Read the model definition and answer for the solid it produces. Units are mm, in the model's axes. A direction names the side the tool comes from. Coordinates: 2 decimals unless noted, no trailing zeros. Write each loop counter-clockwise with the first axis right and the second up, starting at its lowest first coordinate (ties: lowest second). Pieces come first, ordered by that corner, then holes. Notation, with made-up numbers: (-6.5, 45.5) -> (34.5, 45.5) arc R34 ccw to (34.5, 81.5) -> close; hole circle Ø5 at (39.25, 43.25). An arc over 180 degrees is marked (long way). Use CSV: the item, a comma, the result in double quotes.
from build123d import *

# Parameters (mm, degrees)
SKICA1_W                                         = 61
SKICA1_H                                         = 17.5
P_IDAT_VYSUNUT_M1_DEPTH                          = 6
SKICA2_W                                         = 43.1
SKICA2_H                                         = 7.8
P_IDAT_VYSUNUT_M2_DEPTH                          = 20
V_LCOV_ZAHLOUBEN_PRO_M3_ROUBY_S_VNIT_D           = 3.4
V_LCOV_ZAHLOUBEN_PRO_M3_ROUBY_S_VNIT_DEPTH       = 10
V_LCOV_ZAHLOUBEN_PRO_M3_ROUBY_S_VNIT_CBORE_D     = 6.5
V_LCOV_ZAHLOUBEN_PRO_M3_ROUBY_S_VNIT_CBORE_DEPTH = 3.4
V_LCOV_ZAHLOUBEN_PRO_M3_ROUBY_S_VNIT_TIP         = 1.021463052
SKICA5_W                                         = 38.387641765
SKICA5_H                                         = 14.060547141
P_IDAT_VYSUNUT_M3_DEPTH                          = 10
SKICA6_W                                         = 38.387641765
SKICA6_H                                         = 5
P_IDAT_VYSUNUT_M4_DEPTH                          = 1.319108231


with BuildPart() as part:
    # Skica1 → Přidat vysunutím1 (new body)
    with BuildSketch(Plane(origin=(0, 0, 0), x_dir=(1, 0, 0), z_dir=(0, 1, 0))):
        Rectangle(SKICA1_W, SKICA1_H)
    extrude(amount=P_IDAT_VYSUNUT_M1_DEPTH)

    # Skica2 → Přidat vysunutím2 (add)
    with BuildSketch(Plane.XZ):
        with Locations((0, -3.15)):
            Rectangle(SKICA2_W, SKICA2_H)
    extrude(amount=P_IDAT_VYSUNUT_M2_DEPTH)

    # Válcové zahloubení pro M3 šrouby s vnitřním šestihranem1
    with Locations(Plane(origin=(0, 6, 0), x_dir=(1, 0, 0), z_dir=(0, 1, 0))):
        with Locations((-25.25, -3.75), (25.25, -3.75)):
            CounterBoreHole(V_LCOV_ZAHLOUBEN_PRO_M3_ROUBY_S_VNIT_D / 2, V_LCOV_ZAHLOUBEN_PRO_M3_ROUBY_S_VNIT_CBORE_D / 2, V_LCOV_ZAHLOUBEN_PRO_M3_ROUBY_S_VNIT_CBORE_DEPTH, depth=V_LCOV_ZAHLOUBEN_PRO_M3_ROUBY_S_VNIT_DEPTH)
            with Locations((0, 0, -(V_LCOV_ZAHLOUBEN_PRO_M3_ROUBY_S_VNIT_DEPTH + V_LCOV_ZAHLOUBEN_PRO_M3_ROUBY_S_VNIT_TIP / 2))):  # 118° drill point
                Cone(0, V_LCOV_ZAHLOUBEN_PRO_M3_ROUBY_S_VNIT_D / 2, V_LCOV_ZAHLOUBEN_PRO_M3_ROUBY_S_VNIT_TIP, mode=Mode.SUBTRACT)

    # Skica5 → Přidat vysunutím3 (add)
    with BuildSketch(Plane(origin=(0, 6, 0), x_dir=(1, 0, 0), z_dir=(0, 1, 0))):
        with Locations((-1.722409319, -0.400618199)):
            Rectangle(SKICA5_W, SKICA5_H)
    extrude(amount=P_IDAT_VYSUNUT_M3_DEPTH)

    # Skica6 → Přidat vysunutím4 (add)
    with BuildSketch(Plane.XY.offset(7.430891769)):
        with Locations((-1.722409319, 13.5)):
            Rectangle(SKICA6_W, SKICA6_H)
    extrude(amount=P_IDAT_VYSUNUT_M4_DEPTH)


solid = part.part
1. Find the intervals of material crossed by line 1 along Z through (x, y) = (-25.25, 4.75); line 2 along Z through (x, y) = (25.25, 1.2); line 3 along X through (y, z) = (-2, -5.75), in increasing order.
Solutions:
line 1,"z = -8.75 to 0.5, 7 to 8.75"
line 2,"z = -8.75 to 2.05, 5.45 to 8.75"
line 3,"x = -21.55 to 21.55"
2. For a pull along Z with two mould halves and no side action, classify faces 1 (the flat face through (-2, 14, 8.75)), 2 (the flat face through (27, 2.6, 5)), 3 (the flat face through (0, -20, -3)), 4 (the flat face through (0, 3, -8.75)) as pulls with the +Z half, pulls with the -Z half, needs draft (parallel to the pull), parting line crosses it, or undercut.
Solutions:
face 1,"pulls with the +Z half"
face 2,"undercut"
face 3,"needs draft"
face 4,"pulls with the -Z half"
3. A cutting plane is placed at C-C (z = -4.5). Give the vertices of the cut face in (x, y).
Solutions:
outline,"(-30.5, 0) -> (-21.55, 0) -> (-21.55, -20) -> (21.55, -20) -> (21.55, 0) -> (30.5, 0) -> (30.5, 6) -> (17.47, 6) -> (17.47, 16) -> (-20.92, 16) -> (-20.92, 6) -> (-30.5, 6) -> close"
4. A cutting plane is placed at A-A (x = 25.25). Give the vertices of the cut face in (y, z), and give its area (3 significant figures).
Solutions:
outline,"(0, -8.75) -> (6, -8.75) -> (6, 0.5) -> (2.6, 0.5) -> (2.6, 2.05) -> (0, 2.05) -> close; (0, 5.45) -> (2.6, 5.45) -> (2.6, 7) -> (6, 7) -> (6, 8.75) -> (0, 8.75) -> close"
area,"74.1 mm^2"
5. A tool of negligible diameter and unlimited length cuts with its end or side. For faces 5 (the flat face through (17.471, 11, 1)), 6 (the cylindrical face through (22.003, 4.324, 3.607)), 7 (the flat face through (-20.916, 11, 1)), 8 (the flat face through (21.55, -10, -3)), from which of +Z, -Z, +X, -X, +Y, -Y can it reach the whole face along a straight path? Write none if from no direction.
Solutions:
face 5,"+Z, -Z, +X, +Y"
face 6,"+Y"
face 7,"+Z, -Z, -X, +Y"
face 8,"+Z, -Z, +X, -Y"
6. Each of these flat-tipped pins is pushed along its axis until it touches: pin 1 Ø5 at (x, y) = (14.5, 6.5) entering from -Z; pin 2 Ø4 at (x, z) = (-25.25, 3.75) entering from -Y; pin 3 Ø8 at (x, y) = (0, 11) entering from -Z; pin 4 Ø2.5 at (y, z) = (-7.5, -2.5) entering from -X. Where does it stop, or does it pass through?
Solutions:
pin 1,"stops at z = -8.75"
pin 2,"stops at y = 0"
pin 3,"stops at z = -6.63"
pin 4,"stops at x = -21.55"
7. A cutting plane is placed at B-B (x = -12). Give the vertices of the cut face in (y, z).
Solutions:
outline,"(-20, -7.05) -> (0, -7.05) -> (0, -8.75) -> (6, -8.75) -> (6, -6.63) -> (16, -6.63) -> (16, 8.75) -> (11, 8.75) -> (11, 7.43) -> (6, 7.43) -> (6, 8.75) -> (0, 8.75) -> (0, 0.75) -> (-20, 0.75) -> close"
8. A cutting plane is placed at D-D (y = -2.5). Give the vertices of the cut face in (x, z), and give its area (3 significant figures).
Solutions:
outline,"(-21.55, -7.05) -> (21.55, -7.05) -> (21.55, 0.75) -> (-21.55, 0.75) -> close"
area,"336 mm^2"
